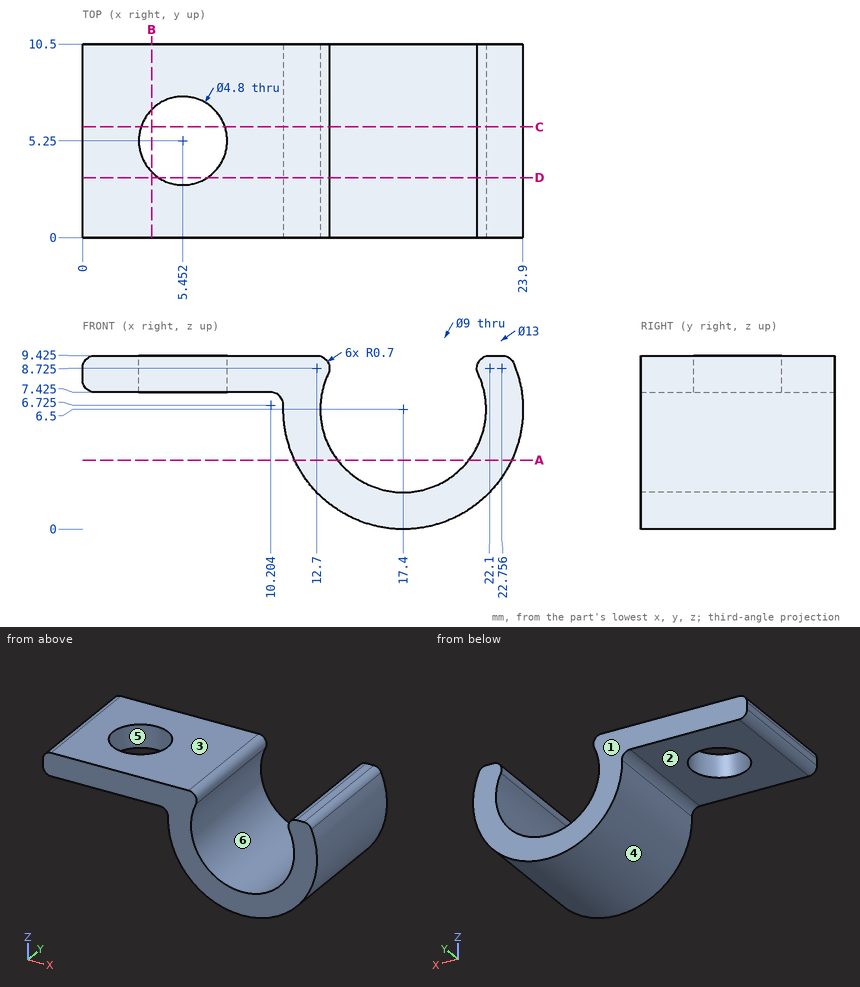
Source: three-view drawing plus pictorial views. Frame: mm from the lowest corner of the part. A direction names the side the tool comes from. Round coordinates to 2 decimals unless told otherwise and drop trailing zeros. Write each loop counter-clockwise with the first axis right and the second up, starting at its lowest first coordinate (ties: lowest second). Pieces come first, ordered by that corner, then holes. Notation, with made-up numbers: M 84.25,-40 L 88.25,-40 A20 ccw 88.25,-17 Z; hole C 59,80.25 d7. An arc over 180 degrees is marked long. Use CSV: the item, a comma, the result in double quotes. Start each with the question number.
Q1. Cut plane A-A on z = 3.75. Output: boundary loops of the cut face in (x, y).
Q2. Cut plane D-D on y = 3.25. Output: boundary loops of the cut face in (x, z) (1 decimal).
Q3. Pull-direction query (X, two-part tool) for the marked faces 3, 4, 5 and 6; classes: +X half, -X half, draft (parallel to the pull), parting line (faces both ways), or undercut.
Q4. Access query for the marked faces 1 and 2. Directions: +Z, -Z, +X, -X, +Y, -Y. A direction counts if a zero-diameter tool reaches every point of the face in a straight line with its end or side. Return the directions, or none.
Q5. Cut plane C-C on y = 6. Output: boundary loops of the cut face in (x, z) (1 decimal).
Q6. Line query: line 1 (X direction, y = 6.5, z = 6.5); line 2 (X direction, y = 7, z = 8) (1 decimal); line 3 (Z direction, x = 17.4, y = 2.5). Output: solid intervals per line, ascending. Write a range as from..to.
Q7. First-contact query: P1, Ø4, axis at x = 5.45, y = 5.25, coming from the +Z side; P2, Ø1.5, axis at y = 6.5, z = 3, coming from the +X side. Flat tips, straight axial feed; report the tip coordinate or a pass-through.
Q8. Cut plane B-B on x = 3.75. Output: boundary loops of the cut face in (y, z) (1 decimal).
Results found:
1,outline,"M 11.51,0 L 13.84,0 L 13.84,10.5 L 11.51,10.5 Z; M 20.96,0 L 23.29,0 L 23.29,10.5 L 20.96,10.5 Z"
2,outline,"M 0,8.1 A0.7 ccw 0.7,7.4 L 4.1,7.4 L 4.1,9.4 L 0.7,9.4 A0.7 ccw 0,8.7 Z; M 6.8,7.4 L 10.2,7.4 A0.7 cw 10.9,6.7 A6.5 ccw long 23.4,9 A0.7 ccw 22.8,9.4 L 22.1,9.4 A0.7 ccw 21.5,8.4 A4.5 cw long 13.3,8.4 A0.7 ccw 12.7,9.4 L 6.8,9.4 Z"
3,face 3,"draft"
3,face 4,"parting line"
3,face 5,"undercut"
3,face 6,"undercut"
4,face 1,"+Z, -Z, +X, -X, +Y"
4,face 2,"-Z, -X, +Y, -Y"
5,outline,"M 0,8.1 A0.7 ccw 0.7,7.4 L 3.2,7.4 L 3.2,9.4 L 0.7,9.4 A0.7 ccw 0,8.7 Z; M 7.7,7.4 L 10.2,7.4 A0.7 cw 10.9,6.7 A6.5 ccw long 23.4,9 A0.7 ccw 22.8,9.4 L 22.1,9.4 A0.7 ccw 21.5,8.4 A4.5 cw long 13.3,8.4 A0.7 ccw 12.7,9.4 L 7.7,9.4 Z"
6,line 1,"10.9..12.9, 21.9..23.9"
6,line 2,"0..3.8, 7.1..13.2, 21.6..23.7"
6,line 3,"0..2"
7,P1,"through"
7,P2,"x = 23.29"
8,outline,"M 0,7.4 L 3.6,7.4 L 3.6,9.4 L 0,9.4 Z; M 6.9,7.4 L 10.5,7.4 L 10.5,9.4 L 6.9,9.4 Z"
